Autodesk Inventor part; units mm, degrees
ref_plane "YZ Plane" through (0, 0, 0) normal (1, 0, 0) x (0, 1, 0)
ref_plane "XZ Plane" through (0, 0, 0) normal (0, 1, 0) x (-1, 0, 0)
ref_plane "XY Plane" through (0, 0, 0) normal (0, 0, 1) x (1, 0, 0)
sketch "Sketch1" plane through (0, 0, 0) normal (0, 0, 1) x (1, 0, 0)
  line L0 (0, 0) -> (15, 0)
  line L1 (15, 0) -> (15, 10)
  line L2 (15, 10) -> (0, 10)
  line L3 (0, 10) -> (0, 0)
  line L4 (1, 9) -> (14, 9)
  line L5 (14, 9) -> (14, 1)
  line L6 (14, 1) -> (1, 1)
  line L7 (1, 1) -> (1, 9)
  dimension "d0" = 15
  dimension "d1" = 10
  dimension "d2" = 13
  dimension "d3" = 8
  dimension "d4" = 1
  dimension "d5" = 1
extrude "Extrusion1" add sketch "Sketch1" along normal blind 20 contours L3 L2 L1 L0 | L4 L5 L6 L7
sketch "Sketch2" plane through (0, 10, 0) normal (0, 1, 0) x (1, 0, 0)
  line L0 (15, 0) -> (0, 0)
  line L1 (0, 0) -> (0, -20)
  line L2 (15, -20) -> (0, -20)
  line L3 (15, 0) -> (15, -20)
  circle A0 centre (5, -5) radius 1.5
  circle A1 centre (5, -15) radius 1.5
  dimension "d8" = 3
  dimension "d9" = 3
  dimension "d10" = 5
  dimension "d11" = 5
  dimension "d12" = 5
  dimension "d13" = 5
extrude "Extrusion2" cut sketch "Sketch2" against normal up to surface (10 mm away) contours A0 | A1
sketch "Sketch3" plane through (15, 0, 0) normal (1, 0, 0) x (0, 0, -1)
  line L0 (0, 0) -> (0, 10)
  line L1 (0, 10) -> (-20, 10)
  line L2 (-20, 0) -> (-20, 10)
  line L3 (0, 0) -> (-20, 0)
  circle A0 centre (-10, 5) radius 1.6
  dimension "d16" = 3.2
  dimension "d17" = 5
  dimension "d18" = 10
extrude "Extrusion3" cut sketch "Sketch3" against normal up to surface (15 mm away) contours A0
properties part number "profile1_3D"
Can you work these out from the model? Positions are in its coordinate system, mm. Coordinates: 2 decimals unless noted, no trailing zeros. Order: outer loops, then holes, each group sorted by start corner. A loop starts at its lowest first (then second) coordinate and runs counter-clockwise, first axis right, second up. Notation, with made-up numbers: M -16,52.25 L -7,52.25 A13 cw -7,69.25 Z; hole C -13,43.5 d7. An arc over 180 degrees is marked long. Answer as CSV lines item,"result".
(1) Suppose I cut it at A-A on x = 5. Please give me the cut outline in (y, z), plus the area to 3 significant figures.
Geometry check:
outline,"M 0,0 L 10,0 L 10,3.5 L 0,3.5 Z; M 0,6.5 L 10,6.5 L 10,13.5 L 0,13.5 Z; M 0,16.5 L 10,16.5 L 10,20 L 0,20 Z; hole C 5,10 d3.2"
area,"132 mm^2"
(2) Please list where these lines run through material, in increasing order: L1, parallel to Z at x = 5, y = 4; L2, parallel to Y at x = 6.5, z = 10; L3, parallel to Z at x = 5.5, y = 3.75.
Geometry check:
L1,"0 to 3.5, 6.5 to 8.75, 11.25 to 13.5, 16.5 to 20"
L2,"0 to 3.4, 6.6 to 10"
L3,"0 to 3.59, 6.41 to 9, 11 to 13.59, 16.41 to 20"
(3) If we mould it in two halves opening along X, with no side actions, what happens to faces 1 (the flat face through (0, 3, 10)), 2 (the flat face through (7, 5, 20)), 3 (the cylindrical face through (6.386, 5.07, 15.575)), 4 (the flat face through (15, 7, 10))? For each: released by +X, released by -X, zero draft, split by the parting line, or undercut.
Geometry check:
face 1,"released by -X"
face 2,"zero draft"
face 3,"undercut"
face 4,"released by +X"
(4) Suppose I cut it at D-D on y = 8.5. Please give me the cut outline in (x, z).
Geometry check:
outline,"M 0,0 L 15,0 L 15,20 L 0,20 Z; hole C 5,5 d3; hole C 5,15 d3"
(5) Suppose I cut it at B-B on z = 10. Please give me the cut outline in (x, y), plus the area to 3 significant figures.
Geometry check:
outline,"M 0,0 L 15,0 L 15,3.4 L 0,3.4 Z; M 0,6.6 L 15,6.6 L 15,10 L 0,10 Z"
area,"102 mm^2"
(6) Suppose I cut it at C-C on y = 4. Please give me the cut outline in (x, z).
Geometry check:
outline,"M 0,0 L 15,0 L 15,8.75 L 0,8.75 Z; M 0,11.25 L 15,11.25 L 15,20 L 0,20 Z; hole C 5,5 d3; hole C 5,15 d3"
